The listing builds one solid part. Answer for the finished solid, in the listing's coordinates (mm). Face numbers are marked on the shaded views. A direction names the side the tool comes from. Round coordinates to 2 decimals unless told otherwise and drop trailing zeros. Order: outer loops, then holes, each group sorted by start corner. A loop starts at its lowest first (then second) coordinate and runs counter-clockwise, first axis right, second up. Notation, with made-up numbers: (47.5, -13.75) -> (84.5, -13.75) arc R20 ccw to (84.5, 1.25) -> close; hole circle Ø6 at (-5, 23.25). An arc over 180 degrees is marked (long way). Return JSON: item names as keys, results as strings. Group by question number.
(1) Which of the six approach directions +Z, -Z, +X, -X, +Y, -Y give full straight-line access (tool end or side, diameter ignored) to the marked faces 1 and 2?
(2) Consider line 1 (X direction, y = 9.5, z = 0); line 2 (X direction, y = 6.25, z = 24); line 3 (Z direction, x = -4, y = 5.25). Determine where each line is inside the solid, lowest interval first. Write a range as [from, to].
(3) The part is cut by section D-D (z = 0). Determine the outline of the cut face in (x, y).
(4) Determine the mould class of the marked faces 3, 4, 5 and 6 for opening direction Z: +Z half, -Z half, draft (parallel to the pull), parting line (faces both ways), or undercut.
(5) The part is cut by section A-A (z = -24). Determine the outline of the cut face in (x, y).
(6) The part is cut by section B-B (y = 10). Determine the outline of the cut face in (x, z), plus the area to 3 significant figures.
(7) Each of these flat-tipped pins is pushed along its axis until it touches: pin 1 (7.5 mm diameter, centred on x = 0, z = -24, fed in from +Y); pin 2 (6 mm diameter, centred on x = 4.5, z = 6, fed in from -Y); pin 3 (4 mm diameter, centred on x = -3, y = 10, fed in from +Z); pin 4 (1.5 mm diameter, centred on x = -8, y = 2.5, fed in from -Z). Where does it stop, or does it pass through?
(8) The part is cut by section C-C (x = -2). Determine the outline of the cut face in (y, z).
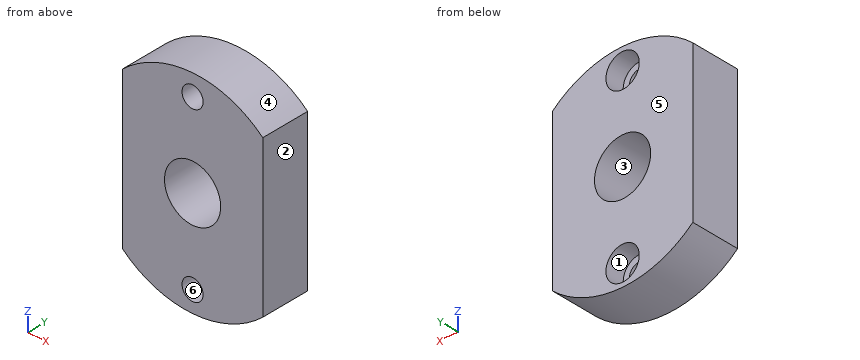
from build123d import *

# Parameters (mm, degrees)
SKETCH_1_R           = 30
EXTRUDE_1_DEPTH      = 14
SKETCH_2_R           = 8
CUT_EXTRUDE_1_DEPTH  = 14
SKETCH_3_R           = 3
CUT_EXTRUDE_2_DEPTH  = 14
SKETCH_4_R           = 4.75
CUT_EXTRUDE_3_DEPTH  = 5.4
SKETCH_5_OUTSIDE_W   = 79.2
SKETCH_5_OUTSIDE_H   = 79.2
SKETCH_5_OUTSIDE_W_2 = 40
SKETCH_5_OUTSIDE_H_2 = 65
CUT_EXTRUDE_4_DEPTH  = 14


with BuildPart() as part:
    # 草图1 → 凸台-拉伸1 (new body)
    with BuildSketch(Plane(origin=(0, 0, 0), x_dir=(1, 0, 0), z_dir=(0, 1, 0))):
        with Locations(Location((0, 0, 0), (0, 0, 270))):
            Circle(SKETCH_1_R)
    extrude(amount=EXTRUDE_1_DEPTH)

    # 草图2 → 切除-拉伸1 (cut)
    with BuildSketch(Plane(origin=(0, 14, 0), x_dir=(1, 0, 0), z_dir=(0, 1, 0))):
        with Locations(Location((0, 0, 0), (0, 0, 270))):
            Circle(SKETCH_2_R)
    extrude(amount=-CUT_EXTRUDE_1_DEPTH, mode=Mode.SUBTRACT)

    # 草图3 → 切除-拉伸2 (cut)
    with BuildSketch(Plane(origin=(0, 14, 0), x_dir=(1, 0, 0), z_dir=(0, 1, 0))):
        with Locations(Location((0, 24, 0), (0, 0, 270))):
            Circle(SKETCH_3_R)
        with Locations(Location((0, -24, 0), (0, 0, 90))):
            Circle(SKETCH_3_R)
    extrude(amount=-CUT_EXTRUDE_2_DEPTH, mode=Mode.SUBTRACT)

    # 草图4 → 切除-拉伸3 (cut)
    with BuildSketch(Plane(origin=(0, 14, 0), x_dir=(1, 0, 0), z_dir=(0, 1, 0))):
        with Locations(Location((0, 24, 0), (0, 0, 270))):
            Circle(SKETCH_4_R)
        with Locations(Location((0, -24, 0), (0, 0, 270))):
            Circle(SKETCH_4_R)
    extrude(amount=-CUT_EXTRUDE_3_DEPTH, mode=Mode.SUBTRACT)

    # 草图5 outside → 切除-拉伸4 (cut)
    with BuildSketch(Plane(origin=(0, 14, 0), x_dir=(1, 0, 0), z_dir=(0, 1, 0))):
        Rectangle(SKETCH_5_OUTSIDE_W, SKETCH_5_OUTSIDE_H)
        Rectangle(SKETCH_5_OUTSIDE_W_2, SKETCH_5_OUTSIDE_H_2, mode=Mode.SUBTRACT)
    extrude(amount=-CUT_EXTRUDE_4_DEPTH, mode=Mode.SUBTRACT)


solid = part.part
Answer below:
{
 "1": {"face 1": "+Y", "face 2": "+Z, -Z, +X, +Y, -Y"},
 "2": {"line 1": "x = [-20, -8], [8, 20]", "line 2": "x = [-18, -3], [3, 18]", "line 3": "z = [-29.73, -6.93], [6.93, 29.73]"},
 "3": {"outline": "(-20, 0) -> (-8, 0) -> (-8, 14) -> (-20, 14) -> close; (8, 0) -> (20, 0) -> (20, 14) -> (8, 14) -> close"},
 "4": {"face 3": "undercut", "face 4": "+Z half", "face 5": "draft", "face 6": "undercut"},
 "5": {"outline": "(-18, 0) -> (-3, 0) -> (-3, 8.6) -> (-4.75, 8.6) -> (-4.75, 14) -> (-18, 14) -> close; (3, 0) -> (18, 0) -> (18, 14) -> (4.75, 14) -> (4.75, 8.6) -> (3, 8.6) -> close"},
 "6": {"outline": "(-20, -22.36) arc R30 ccw to (20, -22.36) -> (20, 22.36) arc R30 ccw to (-20, 22.36) -> close; hole circle Ø16 at (0, 0); hole circle Ø9.5 at (0, -24); hole circle Ø9.5 at (0, 24)", "area": "1,870 mm²"},
 "7": {"pin 1": "stops at y = 8.6", "pin 2": "stops at y = 0", "pin 3": "stops at z = 29.98", "pin 4": "stops at z = -29.11"},
 "8": {"outline": "(0, -29.93) -> (14, -29.93) -> (14, -28.31) -> (8.6, -28.31) -> (8.6, -26.24) -> (0, -26.24) -> close; (0, -21.76) -> (8.6, -21.76) -> (8.6, -19.69) -> (14, -19.69) -> (14, -7.75) -> (0, -7.75) -> close; (0, 7.75) -> (14, 7.75) -> (14, 19.69) -> (8.6, 19.69) -> (8.6, 21.76) -> (0, 21.76) -> close; (0, 26.24) -> (8.6, 26.24) -> (8.6, 28.31) -> (14, 28.31) -> (14, 29.93) -> (0, 29.93) -> close"}
}
